```python
from build123d import *

# Parameters (mm, degrees)
SKETCH1_W           = 28.32
SKETCH1_H           = 25.78
SKETCH1_R           = 1.2
BOSS_EXTRUDE1_DEPTH = 5
SKETCH3_R           = 2.9
CUT_EXTRUDE1_DEPTH  = 0.75
CHAMFER1_SIZE       = 0.5


with BuildPart() as part:
    # Sketch1 → Boss-Extrude1 (new body)
    with BuildSketch(Plane(origin=(0, 0, 0), x_dir=(1, 0, 0), z_dir=(0, 1, 0))):
        Rectangle(SKETCH1_W, SKETCH1_H)
        with Locations((-10.16, 8.89)):
            Circle(SKETCH1_R, mode=Mode.SUBTRACT)
        with Locations((10.16, 8.89)):
            Circle(SKETCH1_R, mode=Mode.SUBTRACT)
        with Locations((10.16, -8.89)):
            Circle(SKETCH1_R, mode=Mode.SUBTRACT)
        with Locations((-10.16, -8.89)):
            Circle(SKETCH1_R, mode=Mode.SUBTRACT)
    extrude(amount=BOSS_EXTRUDE1_DEPTH)

    # Sketch3 → Cut-Extrude1 (cut)
    with BuildSketch(Plane(origin=(0, 5, 0), x_dir=(1, 0, 0), z_dir=(0, 1, 0))):
        with Locations((-10.16, 8.89)):
            Circle(SKETCH3_R)
        with Locations((10.16, 8.89)):
            Circle(SKETCH3_R)
        with Locations((10.16, -8.89)):
            Circle(SKETCH3_R)
        with Locations((-10.16, -8.89)):
            Circle(SKETCH3_R)
    extrude(amount=-CUT_EXTRUDE1_DEPTH, mode=Mode.SUBTRACT)

    # Chamfer1
    chamfer1_edges = [part.edges().sort_by_distance(p)[0] for p in [
        (-11.36, 0, -8.89),
        (8.96, 0, -8.89),
        (8.96, 0, 8.89),
        (-11.36, 0, 8.89),
        (-14.16, 0, 0),
        (0, 0, -12.89),
        (14.16, 0, 0),
        (0, 0, 12.89),
    ]]
    chamfer(chamfer1_edges, length=CHAMFER1_SIZE)


solid = part.part
```
Verification items for the finished model (mm, model axes). A direction names the side the tool comes from. Give positions to 0.01 mm unless a question says otherwise; leave off trailing zeros. Loops run counter-clockwise (first coordinate to the right, second up) from the corner with the lowest first, then second, coordinate; pieces in that order, holes last. Notation, with made-up numbers: M 75.5,28 L 125.5,28 A16 cw 125.5,53 Z; hole C -36,13 d1. An arc over 180 degrees is marked long. Return JSON: item names as keys, results as strings.
1) Section check C-C, the plane y = 3.4. Enter the section's corners in (x, z), and give its area (3 significant figures).
Findings:
{"outline": "M -14.16,-12.89 L 14.16,-12.89 L 14.16,12.89 L -14.16,12.89 Z; hole C -10.16,-8.89 d2.4; hole C -10.16,8.89 d2.4; hole C 10.16,-8.89 d2.4; hole C 10.16,8.89 d2.4", "area": "712 mm2"}
2) Gauge pin test, flat ends, axial feed: P1, Ø7.5, axis at x = -10.16, z = 8.89, coming from the +Y side; P2, Ø1.7, axis at x = 11, z = 10.5, coming from the +Y side; P3, Ø3, axis at x = 10.16, z = 8.89, coming from the -Y side. Record the tip position at first contact, or that the pin passes through.
Findings:
{"P1": "stops at y = 5", "P2": "stops at y = 4.25", "P3": "stops at y = 0.2"}
3) Section check D-D, the plane z = -6.75. Enter the section's corners in (x, y), and give its area (3 significant figures).
Findings:
{"outline": "M -14.16,0.5 L -13.66,0 L 13.66,0 L 14.16,0.5 L 14.16,5 L 12.12,5 L 12.12,4.25 L 8.2,4.25 L 8.2,5 L -8.2,5 L -8.2,4.25 L -12.12,4.25 L -12.12,5 L -14.16,5 Z", "area": "135 mm2"}
4) Section check B-B, the plane z = 8.89. Enter the section's corners in (x, y), and give its area (3 significant figures).
Findings:
{"outline": "M -14.16,0.5 L -13.66,0 L -11.86,0 L -11.36,0.5 L -11.36,4.25 L -13.06,4.25 L -13.06,5 L -14.16,5 Z; M -8.96,0.5 L -8.46,0 L 8.46,0 L 8.96,0.5 L 8.96,4.25 L 7.26,4.25 L 7.26,5 L -7.26,5 L -7.26,4.25 L -8.96,4.25 Z; M 11.36,0.5 L 11.86,0 L 13.66,0 L 14.16,0.5 L 14.16,5 L 13.06,5 L 13.06,4.25 L 11.36,4.25 Z", "area": "112 mm2"}
5) Section check A-A, the plane x = 10.16. Enter the section's corners in (y, z).
Findings:
{"outline": "M 0,-12.39 L 0.5,-12.89 L 5,-12.89 L 5,-11.79 L 4.25,-11.79 L 4.25,-10.09 L 0.5,-10.09 L 0,-10.59 Z; M 0,-7.19 L 0.5,-7.69 L 4.25,-7.69 L 4.25,-5.99 L 5,-5.99 L 5,5.99 L 4.25,5.99 L 4.25,7.69 L 0.5,7.69 L 0,7.19 Z; M 0,10.59 L 0.5,10.09 L 4.25,10.09 L 4.25,11.79 L 5,11.79 L 5,12.89 L 0.5,12.89 L 0,12.39 Z"}
6) Material ranges on L1, parallel to Z at x = -10.16, y = 4.55; L2, parallel to X at y = 2.3, z = -8.89; L3, parallel to X at y = 4.7, z = 8.89, recorded low to high. Write a range as [from, to].
Findings:
{"L1": "z = [-12.89, -11.79], [-5.99, 5.99], [11.79, 12.89]", "L2": "x = [-14.16, -11.36], [-8.96, 8.96], [11.36, 14.16]", "L3": "x = [-14.16, -13.06], [-7.26, 7.26], [13.06, 14.16]"}
7) Mould release check, pull along X, two halves, no side actions. Record for faces 1 (the flat face through (-9, 4.25, -8)), 2 (the flat face through (0, 3, -12.89)), 3 (the cylindrical face through (-10.538, 4.63, 6.015)), 4 (the flat face through (-14.16, 3, 0)): released by +X, released by -X, zero draft, split by the parting line, or undercut.
Findings:
{"face 1": "undercut", "face 2": "zero draft", "face 3": "undercut", "face 4": "released by -X"}
8) Tool access check on faces 5 (the cylindrical face through (-11.36, 2.35, -8.94)), 6 (the flat face through (11, 4.25, 10)). Record the directions out of +Z, -Z, +X, -X, +Y, -Y that give a thin tool (end or side, any length) a straight path to the whole face; none if there is none.
Findings:
{"face 5": "+Y, -Y", "face 6": "+Y"}
